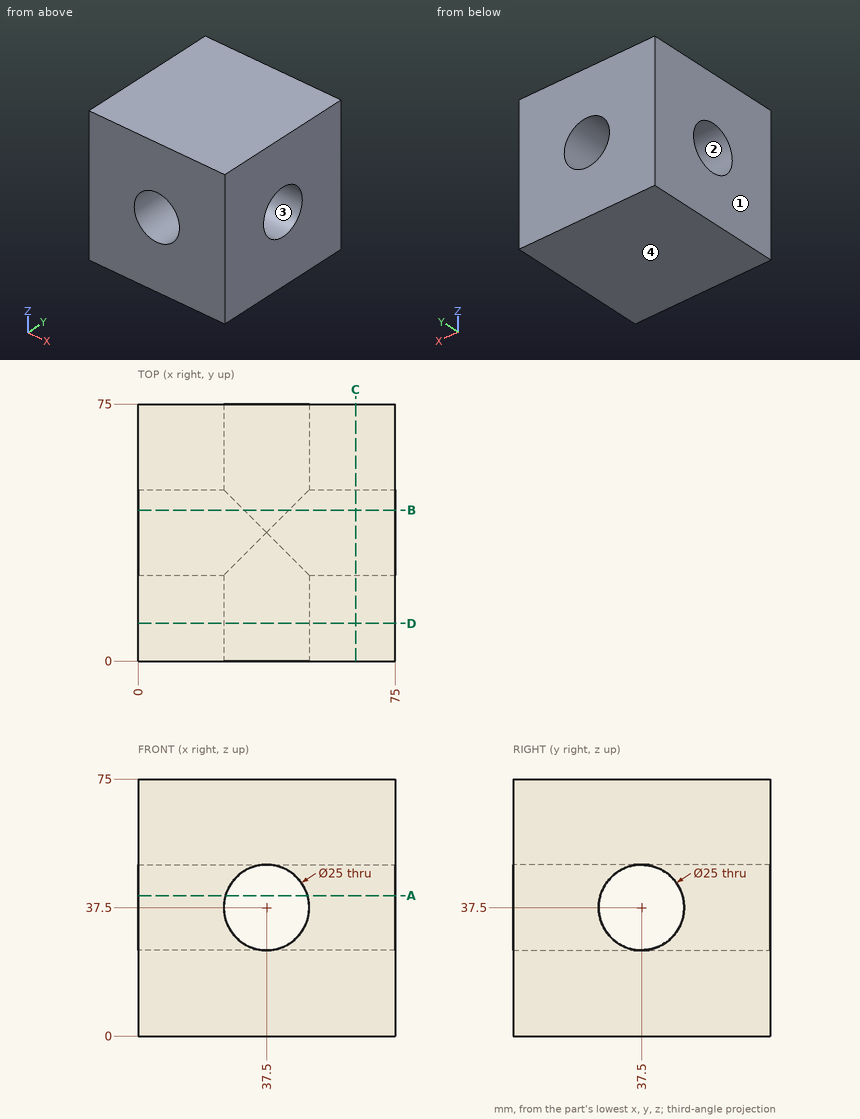
Geometry: see drawing. Coordinates: mm, zero at the bounding-box minimum. Give positions to 0.01 mm unless a question says otherwise; leave off trailing zeros. Order: outer loops, then holes, each group sorted by start corner. A loop starts at its lowest first (then second) coordinate and runs counter-clockwise, first axis right, second up. Notation, with made-up numbers: (-35.5, 75.5) - (14.5, 75.5) arc R23 cw to (14.5, 111.5) - close; hole circle Ø3 at (24, 60). An arc over 180 degrees is marked (long way). Use a Markdown table: item, result.
(1) Pin query (flat end, axial travel): pin 1 (15 mm diameter, centred on x = 37.5, z = 37.5, fed in from +Y). Return the tip coordinate at first contact, or that it passes through.
Computed values:
| item | result |
|---|---|
| pin 1 | passes through |
(2) Section query A-A (z = 41). Output: boundary loops of the cut face in (x, y), then the cut area to 3 significant figures.
Computed values:
| item | result |
|---|---|
| outline | (0, 0) - (25.5, 0) - (25.5, 25.5) - (0, 25.5) - close; (0, 49.5) - (25.5, 49.5) - (25.5, 75) - (0, 75) - close; (49.5, 0) - (75, 0) - (75, 25.5) - (49.5, 25.5) - close; (49.5, 49.5) - (75, 49.5) - (75, 75) - (49.5, 75) - close |
| area | 2,600 mm2 |
(3) Draft query along Z for the marked faces 1, 2, 3 and 4. Return one class per face: released by +Z, released by -Z, zero draft, split by the parting line, or undercut.
Computed values:
| item | result |
|---|---|
| face 1 | zero draft |
| face 2 | undercut |
| face 3 | undercut |
| face 4 | released by -Z |
(4) Section query C-C (x = 63.5). Output: boundary loops of the cut face in (y, z), then the cut area to 3 significant figures.
Computed values:
| item | result |
|---|---|
| outline | (0, 0) - (75, 0) - (75, 75) - (0, 75) - close; hole circle Ø25 at (37.5, 37.5) |
| area | 5,130 mm2 |
(5) Line query: line 1 (X direction, y = 16, z = 37); line 2 (Y direction, x = 61.5, z = 37.5). Output: solid intervals per line, ascending. Write a range as from..to.
Computed values:
| item | result |
|---|---|
| line 1 | x = 0..25.01, 49.99..75 |
| line 2 | y = 0..25, 50..75 |
(6) Section query B-B (y = 44). Output: boundary loops of the cut face in (x, z), then the cut area to 3 significant figures.
Computed values:
| item | result |
|---|---|
| outline | (0, 0) - (75, 0) - (75, 26.82) - (44, 26.82) arc R12.5 cw to (31, 26.82) - (0, 26.82) - close; (0, 48.18) - (31, 48.18) arc R12.5 cw to (44, 48.18) - (75, 48.18) - (75, 75) - (0, 75) - close |
| area | 3,990 mm2 |
